Geometry: final body of the model. Coordinates: model frame, mm. Coordinates: 2 decimals unless noted, no trailing zeros. Order: outer loops, then holes, each group sorted by start corner. A loop starts at its lowest first (then second) coordinate and runs counter-clockwise, first axis right, second up. Notation, with made-up numbers: (39, -22) - (81, -22) arc R36 ccw to (81, 15) - close; hole circle Ø10 at (55.5, 65). An arc over 180 degrees is marked (long way). Use a Markdown table: item, result. Add a question column.
Autodesk Inventor part; units mm, degrees
ref_plane "YZ Plane" through (0, 0, 0) normal (1, 0, 0) x (0, 1, 0)
ref_plane "XZ Plane" through (0, 0, 0) normal (0, 1, 0) x (-1, 0, 0)
ref_plane "XY Plane" through (0, 0, 0) normal (0, 0, 1) x (1, 0, 0)
sketch "スケッチ3" plane through (0, 0, 0) normal (0, 0, 1) x (1, 0, 0)
  circle A0 centre (110.4743, -16.4118) radius 30.1 construction
  circle A1 centre (150.4743, 0.5882) radius 1.5
  circle A2 centre (127.6431, 30.2622) radius 1.5
  circle A3 centre (80.4743, 23.124) radius 1.5
  circle A4 centre (70.4743, -10.4118) radius 1.5
  circle A5 centre (110.4743, -16.4118) radius 7.025
  arc A6 (79.801, 27.5733) -> (76.162, 24.4099) centre (80.4743, 23.124) ccw
  arc A7 (131.2097, 33.0062) -> (126.9698, 34.7115) centre (127.6431, 30.2622) ccw
  arc A8 (154.401, -1.6098) -> (154.0408, 3.3323) centre (150.4743, 0.5882) ccw
  arc A9 (66.162, -9.1259) -> (66.7172, -12.8885) centre (70.4743, -10.4118) ccw
  arc A10 (117.3199, -46.749) -> (137.6119, -31.6026) centre (110.4743, -16.4118) ccw
  line L0 (154.401, -1.6098) -> (137.6119, -31.6026)
  line L1 (66.162, -9.1259) -> (76.162, 24.4099)
  line L2 (79.801, 27.5733) -> (126.9698, 34.7115)
  line L3 (131.2097, 33.0062) -> (154.0408, 3.3323)
  line L4 (96.5433, 16.3458) -> (118.2214, -10.0492) construction
  line L5 (117.0311, -23.9953) -> (91.1935, -46.3348) construction
  circle A11 centre (100.1953, 16.6261) radius 3 construction
  circle A12 centre (144.4932, -10.0968) radius 3 construction
  circle A13 centre (100.1953, 16.6261) radius 4.5 construction
  circle A14 centre (144.4932, -10.0968) radius 4.5 construction
  arc A15 (90.988, -49.7066) -> (95.7356, -51.6195) centre (94.7451, -47.2298) ccw
  circle A16 centre (94.7451, -47.2298) radius 3 construction
  line L6 (95.7356, -51.6195) -> (117.3199, -46.749)
  line L7 (66.7172, -12.8885) -> (90.988, -49.7066)
  circle A17 centre (100.1953, 16.6261) radius 1.25
  circle A18 centre (144.4932, -10.0968) radius 1.25
  circle A19 centre (94.7451, -47.2298) radius 1.25
  circle A20 centre (110.4743, -16.4118) radius 30.1 construction
  circle A21 centre (150.4743, 0.5882) radius 1.5
  circle A22 centre (127.6431, 30.2622) radius 1.5
  circle A23 centre (80.4743, 23.124) radius 1.5
  circle A24 centre (70.4743, -10.4118) radius 1.5
  circle A25 centre (110.4743, -16.4118) radius 7.025
  arc A26 (79.801, 27.5733) -> (76.162, 24.4099) centre (80.4743, 23.124) ccw
  arc A27 (131.2097, 33.0062) -> (126.9698, 34.7115) centre (127.6431, 30.2622) ccw
  arc A28 (154.401, -1.6098) -> (154.0408, 3.3323) centre (150.4743, 0.5882) ccw
  arc A29 (66.162, -9.1259) -> (66.7172, -12.8885) centre (70.4743, -10.4118) ccw
  arc A30 (117.3199, -46.749) -> (137.6119, -31.6026) centre (110.4743, -16.4118) ccw
  line L8 (154.401, -1.6098) -> (137.6119, -31.6026)
  line L9 (66.162, -9.1259) -> (76.162, 24.4099)
  line L10 (79.801, 27.5733) -> (126.9698, 34.7115)
  line L11 (131.2097, 33.0062) -> (154.0408, 3.3323)
  line L12 (96.5433, 16.3458) -> (118.2214, -10.0492) construction
  line L13 (117.0311, -23.9953) -> (91.1935, -46.3348) construction
  circle A31 centre (100.1953, 16.6261) radius 3 construction
  circle A32 centre (144.4932, -10.0968) radius 3 construction
  circle A33 centre (100.1953, 16.6261) radius 4.5 construction
  circle A34 centre (144.4932, -10.0968) radius 4.5 construction
  arc A35 (90.988, -49.7066) -> (95.7356, -51.6195) centre (94.7451, -47.2298) ccw
  circle A36 centre (94.7451, -47.2298) radius 3 construction
  line L14 (95.7356, -51.6195) -> (117.3199, -46.749)
  line L15 (66.7172, -12.8885) -> (90.988, -49.7066)
  circle A37 centre (100.1953, 16.6261) radius 1.25
  circle A38 centre (144.4932, -10.0968) radius 1.25
  circle A39 centre (94.7451, -47.2298) radius 1.25
  circle A40 centre (153.2732, 5.5882) radius 1.5
  circle A41 centre (138.2732, 5.5882) radius 1.5
  arc A42 (157.1998, 3.3902) -> (156.3941, 8.8301) centre (153.2732, 5.5882) ccw
  line L16 (154.401, -1.6098) -> (157.1998, 3.3902)
  line L17 (130.7641, 33.504) -> (156.3941, 8.8301)
  circle A43 centre (138.2732, 5.5882) radius 3
  circle A44 centre (153.2732, 5.5882) radius 3
  point P0 (0, 0)
  point P1 (0, 0)
  point P2 (0, 0)
  dimension "d20" = 14.05
  dimension "d21" = 9
  dimension "d22" = 9
  dimension "d23" = 9
  dimension "d24" = 9
  dimension "d25" = 1
  dimension "d26" = 6
  dimension "d27" = 6
  dimension "d28" = 9
  dimension "d29" = 9
  dimension "d30" = 9
  dimension "d31" = 6
  dimension "d32" = 2.5
  dimension "d33" = 2.5
  dimension "d34" = 2.5
  dimension "d37" = 14.05
  dimension "d38" = 9
  dimension "d39" = 9
  dimension "d40" = 9
  dimension "d41" = 9
  dimension "d42" = 1
  dimension "d43" = 6
  dimension "d44" = 6
  dimension "d45" = 9
  dimension "d46" = 9
  dimension "d47" = 9
  dimension "d48" = 6
  dimension "d49" = 2.5
  dimension "d50" = 2.5
  dimension "d51" = 2.5
  dimension "d52" = 3
  dimension "d53" = 3
  dimension "d54" = 15
  dimension "d55" = 9
  dimension "d56" = 6
  dimension "d57" = 6
  dimension "d58" = 5
extrude "押し出し3" add sketch "スケッチ3" along normal blind 3 contours A1 | L2 A7 L3 A44 A8 L0 A10 L6 A15 L7 A9 L1 A6 | L17 A42 L16 A8 A44 L3 A7 | A44 A8 L3 A40 | L3 A40 A8 A44 | A40 L3 | L3 A40 | A43
extrude "押し出し4" cut sketch "スケッチ3" along normal blind 10 contours A40 L3 | L3 A40
sketch "スケッチ4" plane through (0, 0, 3) normal (0, 0, 1) x (1, 0, 0)
  circle A0 centre (153.2732, 5.5882) radius 1.5
  circle A1 centre (138.2732, 5.5882) radius 1.5
  circle A2 centre (110.4743, -16.4118) radius 7.025
  circle A3 centre (70.4743, -10.4118) radius 1.5
  circle A4 centre (80.4743, 23.124) radius 1.5
  circle A5 centre (127.6431, 30.2622) radius 1.5
  circle A6 centre (94.7451, -47.2298) radius 1.25
  circle A7 centre (144.4932, -10.0968) radius 1.25
  circle A8 centre (100.1953, 16.6261) radius 1.25
  arc A9 (79.801, 27.5733) -> (76.162, 24.4099) centre (80.4743, 23.124) ccw
  line L0 (76.162, 24.4099) -> (66.162, -9.1259)
  arc A10 (66.162, -9.1259) -> (66.7172, -12.8885) centre (70.4743, -10.4118) ccw
  line L1 (66.7172, -12.8885) -> (90.988, -49.7066)
  arc A11 (90.988, -49.7066) -> (95.7356, -51.6195) centre (94.7451, -47.2298) ccw
  line L2 (95.7356, -51.6195) -> (117.3199, -46.749)
  arc A12 (117.3199, -46.749) -> (137.6119, -31.6026) centre (110.4743, -16.4118) ccw
  line L3 (137.6119, -31.6026) -> (157.1998, 3.3902)
  arc A13 (157.1998, 3.3902) -> (156.3941, 8.8301) centre (153.2732, 5.5882) ccw
  line L4 (156.3941, 8.8301) -> (130.7641, 33.504)
  arc A14 (130.7641, 33.504) -> (126.9698, 34.7115) centre (127.6431, 30.2622) ccw
  line L5 (126.9698, 34.7115) -> (79.801, 27.5733)
  circle A15 centre (127.6431, 30.2622) radius 4.025
  arc A16 (131.983, 34.4054) -> (126.5593, 36.1635) centre (127.6431, 30.2622) ccw
  line L6 (79.6614, 27.5499) -> (126.5593, 36.1635)
  line L7 (131.983, 34.4054) -> (156.528, 8.6956)
  point P0 (0, 0)
  dimension "d61" = 8.05
  dimension "d62" = 12
extrude "押し出し5" add sketch "スケッチ4" against normal blind 3 contours A9 L6 A16 L7 A13 L4 A14 L5
extrude "押し出し6" cut sketch "スケッチ4" against normal blind 3 contours A15
sketch "スケッチ5" plane through (0, 0, 3) normal (0, 0, 1) x (1, 0, 0)
  circle A0 centre (127.6431, 30.2622) radius 4.025
  circle A1 centre (153.2732, 5.5882) radius 1.5
  circle A2 centre (138.2732, 5.5882) radius 1.5
  circle A3 centre (110.4743, -16.4118) radius 7.025
  circle A4 centre (70.4743, -10.4118) radius 1.5
  circle A5 centre (80.4743, 23.124) radius 1.5
  circle A6 centre (94.7451, -47.2298) radius 1.25
  circle A7 centre (144.4932, -10.0968) radius 1.25
  circle A8 centre (100.1953, 16.6261) radius 1.25
  arc A9 (79.6614, 27.5499) -> (76.162, 24.4099) centre (80.4743, 23.124) ccw
  line L0 (76.162, 24.4099) -> (66.162, -9.1259)
  arc A10 (66.162, -9.1259) -> (66.7172, -12.8885) centre (70.4743, -10.4118) ccw
  line L1 (66.7172, -12.8885) -> (90.988, -49.7066)
  arc A11 (90.988, -49.7066) -> (95.7356, -51.6195) centre (94.7451, -47.2298) ccw
  line L2 (95.7356, -51.6195) -> (117.3199, -46.749)
  arc A12 (117.3199, -46.749) -> (137.6119, -31.6026) centre (110.4743, -16.4118) ccw
  line L3 (137.6119, -31.6026) -> (157.1998, 3.3902)
  arc A13 (157.1998, 3.3902) -> (156.528, 8.6956) centre (153.2732, 5.5882) ccw
  line L4 (156.528, 8.6956) -> (131.983, 34.4054)
  arc A14 (131.983, 34.4054) -> (126.5593, 36.1635) centre (127.6431, 30.2622) ccw
  line L5 (126.5593, 36.1635) -> (79.6614, 27.5499)
  circle A15 centre (153.2732, 5.5882) radius 2
  circle A16 centre (138.2732, 5.5882) radius 2
  arc A17 (157.6055, 3.092) -> (156.8408, 9.0914) centre (153.2732, 5.5882) ccw
  line L6 (131.9243, 34.466) -> (156.8408, 9.0914)
  line L7 (157.6055, 3.092) -> (137.4212, -31.9384)
  arc A18 (117.3199, -46.749) -> (137.6119, -31.6026) centre (110.4743, -16.4118) ccw
  arc A19 (131.983, 34.4054) -> (126.5593, 36.1635) centre (127.6431, 30.2622) ccw
  point P0 (0, 0)
  dimension "d67" = 4
  dimension "d68" = 4
  dimension "d69" = 3
extrude "押し出し7" add sketch "スケッチ5" against normal blind 3 contours L6 A17 L7 A12 L3 A13 L4
extrude "押し出し8" cut sketch "スケッチ5" against normal blind 3 contours A15 | A16
properties part number "前足内フレーム" material "アルミニウム 2014-T4"
1) Section query C-C (z = 2.3). Give the number of separate pieces and of enclosed holes in the cut face, and give its area (3 significant figures).
2) Section query A-A (x = 108). Return the cut outline in (y, z).
3) Line query: line 1 (X direction, y = -16.5, z = 2.85); line 2 (X direction, y = -17.5, z = 1.6); line 3 (X direction, y = 1.5, z = 0.8). Output: solid intervals per line, ascending. Write a range as from..to.
4) Section query D-D (y = -30.5). Return the cut outline in (x, z), and give its area (3 significant figures).
5) First-contact query: pin 1 (4.5 mm diameter, centred on x = 138.27, y = 5.59, fed in from +Z); pin 2 (1.5 mm diameter, centred on x = 130.5, z = 0.5, fed in from +Y); pin 3 (1.5 mm diameter, centred on x = 85.5, z = 0.5, fed in from -Y); pin 4 (1 mm diameter, centred on x = 133, z = 2.5, fed in from +Y). Flat tips, straight axial feed; report the tip coordinate or a pass-through.
6) Section query B-B (y = -21.5). Return the cut outline in (x, z), and give its area (3 significant figures).
7) Draft query along Y for faces 1 (the cylindrical face through (143.244, -10.152, 1.479)), 2 (the cylindrical face through (140.12, 4.82, 1.52)), 3 (the flat face through (147.655, -14.178, 1.521)), 4 (the flat face through (71.092, 7.407, 1.479)). Return one class per face: released by +Y, released by -Y, zero draft, split by the parting line, or undercut.
From the geometry:
| question | item | result |
|---|---|---|
| 1 | separate pieces | 1 |
| 1 | enclosed holes | 9 |
| 1 | area | 5,340 mm^2 |
| 2 | outline | (-48.85, 0) - (-22.99, 0) - (-22.99, 3) - (-48.85, 3) - close; (-9.84, 0) - (32.75, 0) - (32.75, 3) - (-9.84, 3) - close |
| 3 | line 1 | x = 69.1..103.45, 117.5..146.32 |
| 3 | line 2 | x = 69.76..103.53, 117.41..145.74 |
| 3 | line 3 | x = 69.33..156.69 |
| 4 | outline | (78.33, 0) - (138.25, 0) - (138.25, 3) - (78.33, 3) - close |
| 4 | area | 180 mm^2 |
| 5 | pin 1 | stops at z = 3 |
| 5 | pin 2 | stops at y = 35.88 |
| 5 | pin 3 | stops at y = -42.52 |
| 5 | pin 4 | stops at y = 33.88 |
| 6 | outline | (72.39, 0) - (105.63, 0) - (105.63, 3) - (72.39, 3) - close; (115.32, 0) - (143.44, 0) - (143.44, 3) - (115.32, 3) - close |
| 6 | area | 184 mm^2 |
| 7 | face 1 | undercut |
| 7 | face 2 | undercut |
| 7 | face 3 | released by -Y |
| 7 | face 4 | released by +Y |
